Input: part model. Units: mm. Frame: model coordinates. Face numbers are marked on the shaded views. Round coordinates to 2 decimals unless told otherwise and drop trailing zeros. Write each loop counter-clockwise with the first axis right and the second up, starting at its lowest first coordinate (ties: lowest second). Pieces come first, ordered by that corner, then holes. Notation, with made-up numbers: (69, 65.25) -> (105, 65.25) arc R25 ccw to (105, 92.25) -> close; hole circle Ø10 at (9, 6). An arc over 180 degrees is marked (long way). Write item = value, one per line.
```python
from build123d import *

# Parameters (mm, degrees)
F2_W            = 25
F2_H            = 76.3443418741
F3_REACH        = 140.3344210413
F3_COPIES_COUNT = 8
F5_W            = 25
F5_H            = 76.3443418741
F6_REACH        = 215.3344210413
F6_COPIES_COUNT = 10


# Not quite as in the source:
# - a pattern or mirror of a feature is missing from the dataset's text; its kind, count and spacing are read off the source's solid


with BuildPart() as f1:
    # F0 (on Front) → F1 (revolve)
    with BuildSketch(Plane.XZ):
        with BuildLine():
            Line((0, 5), (0, 0))
            Line((0, 0), (60, 0))
            Line((60, 0), (60, 96))
            Line((60, 96), (55, 96))
            Line((55, 96), (55, 5))
            Line((55, 5), (50, 5))
            Line((50, 5), (50, 96))
            Line((50, 96), (45, 96))
            Line((45, 96), (45, 10))
            ThreePointArc((45, 10), (43.5355339059, 6.4644660941), (40, 5))
            Line((40, 5), (0, 5))
        make_face()
    revolve(axis=Axis((0, 0, 2.5), (0, 0, 1)))

    f3_end = f1.faces().sort_by_distance((-50, 0, 50.5))[0]
    # F2 (on Front) → F3 (cut, up to a face of the model that its end follows)
    with BuildSketch(Plane.XZ):
        with Locations((0, 48)):
            Rectangle(F2_W, F2_H)
    f3_long = extrude(amount=F3_REACH, mode=Mode.PRIVATE)
    f3 = split(f3_long, bisect_by=f3_end, keep=Keep.BOTTOM, mode=Mode.PRIVATE)
    add(f3, mode=Mode.SUBTRACT)

    # F3_copies: F3 ×8 about axis
    f3_copies_axis = Axis((0, 0, 0), (0, 0, 1))
    for i in range(1, F3_COPIES_COUNT):
        add(f3.rotate(f3_copies_axis, i * 360 / F3_COPIES_COUNT), mode=Mode.SUBTRACT)

    f6_end = f1.faces().sort_by_distance((-55, 0, 50.5))[0]
    # F5 (on offset) → F6 (cut, up to a face of the model that its end follows)
    with BuildSketch(Plane.XZ.offset(75)):
        with Locations((0, 48)):
            Rectangle(F5_W, F5_H)
    f6_long = extrude(amount=-F6_REACH, mode=Mode.PRIVATE)
    f6 = split(f6_long, bisect_by=f6_end, keep=Keep.ALL, mode=Mode.PRIVATE).solids().sort_by_distance((0, -75, 48))[0]
    add(f6, mode=Mode.SUBTRACT)

    # F6_copies: F6 ×10 about axis
    f6_copies_axis = Axis((0, 0, 0), (0, 0, 1))
    for i in range(1, F6_COPIES_COUNT):
        add(f6.rotate(f6_copies_axis, i * 360 / F6_COPIES_COUNT), mode=Mode.SUBTRACT)


solid = f1.part
```
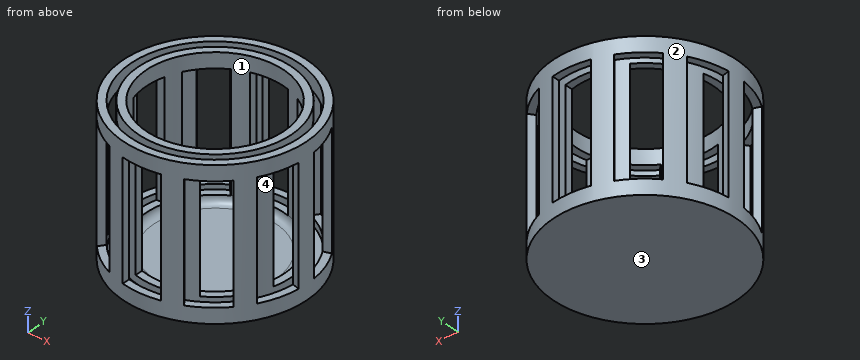
1) Line query: L1, parallel to Y at x = 0.5, z = 89; L2, parallel to X at y = -0.5, z = 21.5; L3, parallel to Z at x = 46, y = 6.5. Output: solid intervals per line, ascending. Write a range as from..to.
Solutions:
L1 = -60..-55, -50..-45, 45..50, 55..60
L2 = -60..-55, 55..60
L3 = 0..9.83, 86.17..96
2) Cut plane B-B (y = 0). Return the cut outline in (x, z), and give its area (3 significant figures).
Solutions:
outline = (-60, 0) -> (60, 0) -> (60, 96) -> (55, 96) -> (55, 5) -> (50, 5) -> (50, 9.83) -> (45, 9.83) arc R5 cw to (40, 5) -> (-40, 5) arc R5 cw to (-45, 9.83) -> (-50, 9.83) -> (-50, 5) -> (-55, 5) -> (-55, 96) -> (-60, 96) -> close; (-50, 86.17) -> (-45, 86.17) -> (-45, 96) -> (-50, 96) -> close; (45, 86.17) -> (50, 86.17) -> (50, 96) -> (45, 96) -> close
area = 1,670 mm^2
3) Cut plane A-A (x = 0). Count the separate pieces of the cut face and the enclosed holes in it, and give its area (3 significant figures).
Solutions:
separate_pieces = 5
enclosed_holes = 0
area = 904 mm^2
4) First-contact query: P1, Ø1.5, axis at x = 25, z = 84, coming from the -Y side; P2, Ø5, axis at x = 44, z = 36, coming from the +Y side; P3, Ø1.6, axis at y = 45.5, z = 50, coming from the -X side. Flat tips, straight axial feed; report the tip coordinate or a pass-through.
Solutions:
P1 = -54.88
P2 = 40.13
P3 = -22.4
5) Draft query along X for the marked faces 1, 2, 3 and 4. Return one class per face: +X half, -X half, draft (parallel to the pull), parting line (faces both ways), or undercut.
Solutions:
face_1 = undercut
face_2 = parting line
face_3 = draft
face_4 = undercut
